```python
from build123d import *

# Parameters (mm, degrees)
BOSS_EXTRU_1_DEPTH      = 75
ESQUISSE2_R             = 5
ENL_V_MAT_EXTRU_1_DEPTH = 75


with BuildPart() as part:
    # Esquisse1 → Boss.-Extru.1 (new body)
    with BuildSketch(Plane.XY):
        with BuildLine():
            Line((-20.64171123, -0.577540107), (-20.64171123, 13.422459893))
            ThreePointArc((-20.64171123, 13.422459893), (-0.64171123, 33.422459893), (19.35828877, 13.422459893))
            Line((19.35828877, 13.422459893), (19.35828877, -0.577540107))
            ThreePointArc((19.35828877, -0.577540107), (17.600929457, -4.820180794), (13.35828877, -6.577540107))
            Line((13.35828877, -6.577540107), (-14.64171123, -6.577540107))
            ThreePointArc((-14.64171123, -6.577540107), (-18.884351917, -4.820180794), (-20.64171123, -0.577540107))
        make_face()
        with BuildLine():
            Line((13.35828877, -2.577540107), (-14.64171123, -2.577540107))
            ThreePointArc((-14.64171123, -2.577540107), (-16.055924792, -1.991753669), (-16.64171123, -0.577540107))
            Line((-16.64171123, -0.577540107), (-16.64171123, 13.422459893))
            ThreePointArc((-16.64171123, 13.422459893), (-0.64171123, 29.422459893), (15.35828877, 13.422459893))
            Line((15.35828877, 13.422459893), (15.35828877, -0.577540107))
            ThreePointArc((15.35828877, -0.577540107), (14.772502332, -1.991753669), (13.35828877, -2.577540107))
        make_face(mode=Mode.SUBTRACT)
    extrude(amount=BOSS_EXTRU_1_DEPTH)

    # Esquisse2 → Enlèv. mat.-Extru.1 (cut)
    with BuildSketch(Plane(origin=(0, 0, 0), x_dir=(1, 0, 0), z_dir=(0, 1, 0))):
        with Locations(Location((-0.64171123, -12.5, 0), (0, 0, 90))):
            Circle(ESQUISSE2_R)
        with Locations(Location((-0.64171123, -62.5, 0), (0, 0, 90))):
            Circle(ESQUISSE2_R)
    extrude(amount=ENL_V_MAT_EXTRU_1_DEPTH, mode=Mode.SUBTRACT)


solid = part.part
```
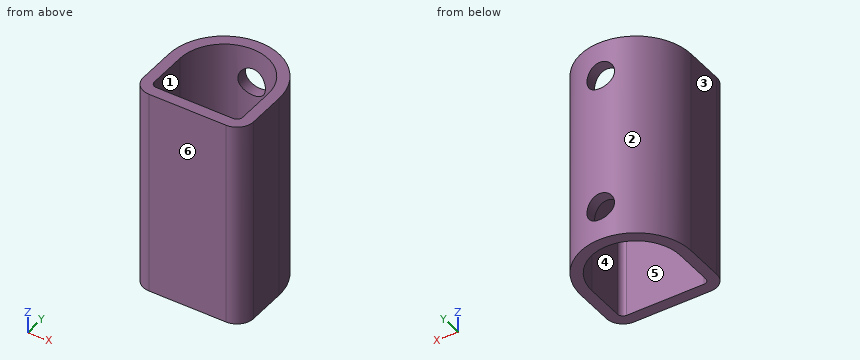
Source: CAD feature listing. Evaluate the final solid. Frame: model axes, mm. Face numbers are marked on the shaded views. A direction names the side the tool comes from. Coordinates: 2 decimals unless noted, no trailing zeros. Write each loop counter-clockwise with the first axis right and the second up, starting at its lowest first coordinate (ties: lowest second). Pieces come first, ordered by that corner, then holes. Notation, with made-up numbers: M 7,-39.5 L 36,-39.5 A28 ccw 36,-11.5 Z; hole C 10,88 d7. An arc over 180 degrees is marked long. Answer as a JSON object with one key per item and string values.
1. Cut plane D-D on z = 12.5. Output: boundary loops of the cut face in (x, y), plus the area to 3 significant figures.
Evaluation:
{"outline": "M -20.64,-0.58 A6 ccw -14.64,-6.58 L 13.36,-6.58 A6 ccw 19.36,-0.58 L 19.36,13.42 A20 ccw 4.36,32.79 L 4.36,28.62 A16 cw 15.36,13.42 L 15.36,-0.58 A2 cw 13.36,-2.58 L -14.64,-2.58 A2 cw -16.64,-0.58 L -16.64,13.42 A16 cw -5.64,28.62 L -5.64,32.79 A20 ccw -20.64,13.42 Z", "area": "460 mm^2"}
2. Cut plane C-C on x = 14.5. Output: boundary loops of the cut face in (y, z).
Evaluation:
{"outline": "M -6.47,0 L -2.22,0 L -2.22,75 L -6.47,75 Z; M 18.59,0 L 26.49,0 L 26.49,75 L 18.59,75 Z"}
3. Access query for the marked faces 1 and 2. Directions: +Z, -Z, +X, -X, +Y, -Y. A direction counts if a zero-diameter tool reaches every point of the face in a straight line with its end or side. Return the directions, or none.
Evaluation:
{"face 1": "+Z, -Z", "face 2": "+Z, -Z, +Y"}
4. Ray query, L1, parallel to X at y = 4, z = 68.5; L2, parallel to Y at x = -1, z = 51.5; L3, parallel to X at y = 27, z = 54. Return the intervals inside material, ascending.
Evaluation:
{"L1": "-20.64 to -16.64, 15.36 to 19.36", "L2": "-6.58 to -2.58, 29.42 to 33.42", "L3": "-15.33 to -9.11, 7.82 to 14.04"}
5. Contact query for flat-ended pins moving along their axis: P1, Ø4, axis at y = 27, z = 9, coming from the +X side; P2, Ø12, axis at y = 27, z = 27.5, coming from the +X side; P3, Ø5, axis at x = 6, z = 46, coming from the +Y side. Output: stop coordinate, or through.
Evaluation:
{"P1": "x = 15.67", "P2": "x = 17.87", "P3": "y = 32.99"}
6. Cut plane A-A on y = 1. Output: boundary loops of the cut face in (x, z), plus the area to 3 significant figures.
Evaluation:
{"outline": "M -20.64,0 L -16.64,0 L -16.64,75 L -20.64,75 Z; M 15.36,0 L 19.36,0 L 19.36,75 L 15.36,75 Z", "area": "600 mm^2"}
7. Cut plane B-B on z = 33. Output: boundary loops of the cut face in (x, y).
Evaluation:
{"outline": "M -20.64,-0.58 A6 ccw -14.64,-6.58 L 13.36,-6.58 A6 ccw 19.36,-0.58 L 19.36,13.42 A20 ccw -20.64,13.42 Z; hole M -16.64,-0.58 A2 ccw -14.64,-2.58 L 13.36,-2.58 A2 ccw 15.36,-0.58 L 15.36,13.42 A16 ccw -16.64,13.42 Z"}
8. Draft query along Y for the marked faces 3, 4, 5 and 6. Return one class per face: released by +Y, released by -Y, zero draft, split by the parting line, or undercut.
Evaluation:
{"face 3": "zero draft", "face 4": "undercut", "face 5": "undercut", "face 6": "released by -Y"}
